Can you work these out from the model? Positions are in its coordinate system, mm. Face numbers are marked on the shaded views. A direction names the side the tool comes from. Give positions to 0.01 mm unless a question says otherwise; leave off trailing zeros. Order: outer loops, then holes, each group sorted by start corner. A loop starts at its lowest first (then second) coordinate and runs counter-clockwise, first axis right, second up.
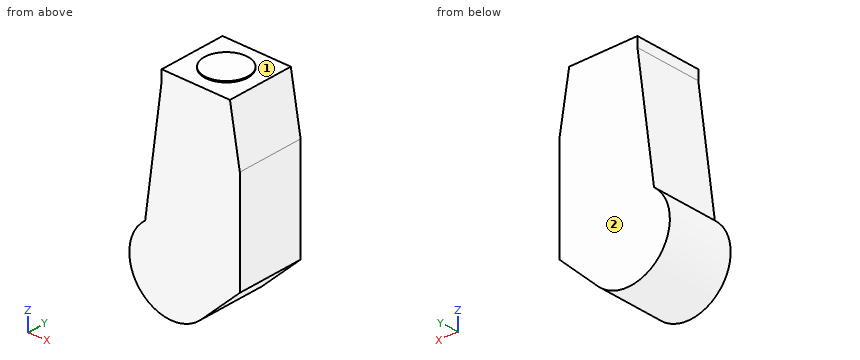
```python
from build123d import *

# Parameters (mm, degrees)
BOSS_EXTRUDE1_DEPTH   = 58
SKETCH2_R             = 37.5
BOSS_EXTRUDE2_DEPTH   = 2
BODY_MOVE_COPY2_ANGLE = 120


with BuildPart() as part:
    # Sketch1 → Boss-Extrude1 (new, symmetric)
    with BuildSketch(Plane.XY):
        with BuildLine():
            Line((291, 0), (291, 17))
            Line((291, 17), (274, 17))
            Line((274, 17), (57, 45.607017004))
            ThreePointArc((57, 45.607017004), (-48.32227677, 54.71706834), (-52.304922539, -50.92342367))
            Line((-52.304922539, -50.92342367), (13, -118))
            Line((13, -118), (191, -118))
            Line((191, -118), (291, -101))
            Line((291, -101), (291, 0))
        make_face()
    extrude(amount=BOSS_EXTRUDE1_DEPTH, both=True)

    # Sketch2 → Boss-Extrude2 (add)
    with BuildSketch(Plane(origin=(291, 0, 0), x_dir=(0, 0, -1), z_dir=(1, 0, 0))):
        with Locations((0, -42)):
            Circle(SKETCH2_R)
    extrude(amount=BOSS_EXTRUDE2_DEPTH)


with BuildPart() as part_1:
    # Body-Move/Copy1: moved
    add(part.part.moved(Location((-293, 42, 0))))


with BuildPart() as part_2:
    # Body-Move/Copy2: moved
    add(part_1.part.rotate(Axis((0, 0, 0), (0.5773502691896272, -0.5773502691896252, 0.5773502691896252)), BODY_MOVE_COPY2_ANGLE))


solid = part_2.part
```
1) Suppose I cut it at C-C (z = -68). Please give me the cut outline in (x, y), and give its area (3 significant figures).
2) Suppose I cut it at B-B (x = -5). Please give me the cut outline in (y, z), and give its area (3 significant figures).
3) Which directions (+Z, -Z, +X, -X, +Y, -Y) give clear straight access to the entire face, cutting with the end or side of a thin tool? Please do the marked faces 1 and 2.
4) I'm going to push flat-ended pins straight in: pin 1 Ø12 at (x, y) = (-52.5, -20.5) entering from -Z; pin 2 Ø1 at (x, y) = (47.5, -19) entering from +Z; pin 3 Ø5 at (y, z) = (-16.5, -6.5) entering from -X. Where does each tip first touch, or does it pass through?
5) Suppose I cut it at A-A (y = 0). Please give me the cut outline in (x, z).
6) If I drill on line 1 (Z direction, x = 9, y = 49.5); line 2 (Z direction, x = -43, y = -37.5); line 3 (X direction, y = 25.5, z = -333), over which ranges is the centre line in solid material (lowest first)?
7) Suppose I cut it at D-D (y = 25). Please give me the cut outline in (x, z).
Results:
1. outline: (-65.46, -58) - (70.22, -58) - (70.22, 58) - (-65.46, 58) - close
1. area: 15,700 mm2
2. outline: (-58, -355.93) - (58, -355.93) - (58, -2) - (37.17, -2) - (37.17, 0) - (-37.17, 0) - (-37.17, -2) - (-58, -2) - close
2. area: 41,200 mm2
3. face 1: +Z
3. face 2: +Z, -Z, +X, -X, +Y
4. pin 1: stops at z = -365.86
4. pin 2: stops at z = -2
4. pin 3: stops at x = -59
5. outline: (-87.61, -236) arc R73 ccw (long way) to (8.92, -345.3) - (76, -280) - (76, -102) - (59, -2) - (37.5, -2) - (37.5, 0) - (-37.5, 0) - (-37.5, -2) - (-59, -2) - (-59, -19) - close
6. line 1: z = -345.23 to -2
6. line 2: z = -365.99 to -2
6. line 3: x = -103.07 to 21.56
7. outline: (-87.61, -236) arc R73 ccw (long way) to (8.92, -345.3) - (76, -280) - (76, -102) - (59, -2) - (27.95, -2) - (27.95, 0) - (-27.95, 0) - (-27.95, -2) - (-59, -2) - (-59, -19) - close
